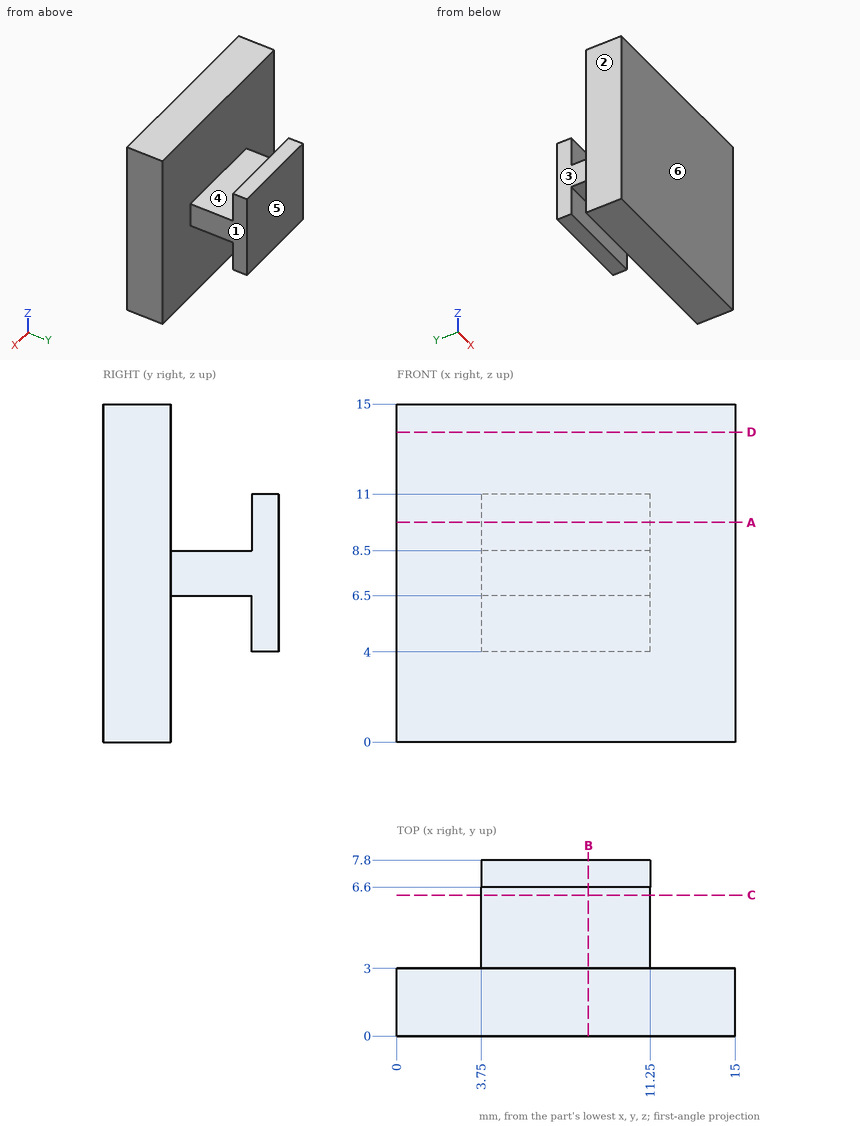
Verification items for this drawing (mm, ordinates from the low corner). A direction names the side the tool comes from. Coordinates: 2 decimals unless noted, no trailing zeros. Write each loop counter-clockwise with the first axis right and the second up, starting at its lowest first coordinate (ties: lowest second). Pieces come first, ordered by that corner, then holes. Notation, with made-up numbers: M 77.5,11 L 95.5,11 A20 ccw 95.5,16 Z; hole C 72.25,50 d5. An arc over 180 degrees is marked long. Answer as a JSON object with one key per item and string values. Group by question number.
(1) Cross-section at C-C, the plane y = 6.25. Record the cut outline in (x, z).
(2) Material ranges on line 1 (Y direction, x = 10, z = 9); line 2 (Y direction, x = 4, z = 2); line 3 (Z direction, x = 4.25, y = 4.25), recorded low to high.
(3) Cross-section at D-D, the plane z = 13.75. Record the cut outline in (x, y), and give its area (3 significant figures).
(4) Cross-section at A-A, the plane z = 9.75. Record the cut outline in (x, y).
(5) Tool access check on the marked faces 1, 2 and 3. Record the directions out of +Z, -Z, +X, -X, +Y, -Y that give a thin tool (end or side, any length) a straight path to the whole face; none if there is none.
(6) Release check for a two-part mould opening along Y. For the marked faces 4, 5 and 6 record: +Y half, -Y half, draft (parallel to the pull), parting line (faces both ways), or undercut.
(7) Cross-section at B-B, the plane x = 8.5. Record the cut outline in (y, z).
(8) Gauge pin test, flat ends, axial feed: pin 1 (2 mm diameter, centred on x = 9, z = 10, fed in from -Y); pin 2 (1 mm diameter, centred on x = 7, y = 7.5, fed in from -Z); pin 3 (1.8 mm diameter, centred on x = 6.5, y = 4, fed in from -Z); pin 4 (1.3 mm diameter, centred on x = 7.5, y = 7, fed in from +Z). Record the tip position at first contact, or that the pin passes through.
Reply:
{
 "1": {"outline": "M 3.75,6.5 L 11.25,6.5 L 11.25,8.5 L 3.75,8.5 Z"},
 "2": {"line 1": "0 to 3, 6.6 to 7.8", "line 2": "0 to 3", "line 3": "6.5 to 8.5"},
 "3": {"outline": "M 0,0 L 15,0 L 15,3 L 0,3 Z", "area": "45.0 mm²"},
 "4": {"outline": "M 0,0 L 15,0 L 15,3 L 0,3 Z; M 3.75,6.6 L 11.25,6.6 L 11.25,7.8 L 3.75,7.8 Z"},
 "5": {"face 1": "+Z, -Z, +X, +Y", "face 2": "+Z, -Z, -X, +Y, -Y", "face 3": "+Z, -Z, -X, +Y"},
 "6": {"face 4": "undercut", "face 5": "+Y half", "face 6": "-Y half"},
 "7": {"outline": "M 0,0 L 3,0 L 3,6.5 L 6.6,6.5 L 6.6,4 L 7.8,4 L 7.8,11 L 6.6,11 L 6.6,8.5 L 3,8.5 L 3,15 L 0,15 Z"},
 "8": {"pin 1": "y = 0", "pin 2": "z = 4", "pin 3": "z = 6.5", "pin 4": "z = 11"}
}
